Read the model definition and answer for the solid it produces. Units are mm, in the model's axes. A direction names the side the tool comes from. Coordinates: 2 decimals unless noted, no trailing zeros. Loops run counter-clockwise (first coordinate to the right, second up) from the corner with the lowest first, then second, coordinate; pieces in that order, holes last. Notation, with made-up numbers: M 40.5,18.5 L 79.5,18.5 A20 ccw 79.5,55.5 Z; hole C 0.25,15 d8. An arc over 180 degrees is marked long. One line per item, written item: value. Start each with the question number.
```python
from build123d import *

# Parameters (mm, degrees)
CROQUIS3_R            = 2.49
CORTAR_EXTRUIR1_DEPTH = 18
CROQUIS4_R            = 1.5
CORTAR_EXTRUIR2_DEPTH = 3


with BuildPart() as part:
    # Croquis2 → Revolución1 (revolve)
    with BuildSketch(Plane.XY, mode=Mode.PRIVATE) as revoluci_n1_sk:
        Polygon((0, 0), (-6, 0), (-6, 2), (-5, 2), (-5, 18), (-6, 18), (-6, 20), (0, 20), align=None)
    revolve(revoluci_n1_sk.sketch.rotate(Axis((0, 0, 0), (0, 1, 0)), 270), axis=Axis((0, 0, 0), (0, 1, 0)))

    # Croquis3 → Cortar-Extruir1 (cut)
    with BuildSketch(Plane.XZ):
        with Locations(Location((0, 0, 0), (0, 0, 270))):
            Circle(CROQUIS3_R)
    extrude(amount=-CORTAR_EXTRUIR1_DEPTH, mode=Mode.SUBTRACT)

    # Croquis4 → Cortar-Extruir2 (cut)
    with BuildSketch(Plane(origin=(5, 0, 0), x_dir=(0, 0, -1), z_dir=(1, 0, 0))):
        with Locations((0, 10)):
            Circle(CROQUIS4_R)
    extrude(amount=-CORTAR_EXTRUIR2_DEPTH, mode=Mode.SUBTRACT)


solid = part.part
```
1) Section B-B (z = 5.25) is taken. Determine the outline of the cut face in (x, y).
2) Flat-ended cylindrical pins translate along their axes: pin 1 (3 mm diameter, centred on y = 12.5, z = 3, fed in from -X); pin 2 (5 mm diameter, centred on y = 10.5, z = 2.5, fed in from +X); pin 3 (2.5 mm diameter, centred on y = 10, z = 0, fed in from +X). Find the tip coordinate at first contact, or state that the pin passes through.
3) A tool of negligible diameter and unlimited length cuts with its end or side. For faces 4 (the face through (0, 18, 0)), 5 (the face through (-1.802, 19.014, -5.723)), 6 (the face through (-4, 10, -3)), 7 (the face through (3.5, 9.1, 1.2)), from which of +Z, -Z, +X, -X, +Y, -Y can it reach the whole face along a straight path? Write none if from no direction.
4) Section D-D (z = 0) is taken. Determine the outline of the cut face in (x, y).
5) Consider line 1 along Y through (x, z) = (3.05, 0); line 2 along Y through (x, z) = (5, -1.5); line 3 along X through (y, z) = (6, 0). Determine where each line is inside the solid, lowest interval first.
6) Section A-A (x = 0) is taken. Determine the outline of the cut face in (y, z).
7) Section C-C (y = 5.25) is taken. Determine the outline of the cut face in (x, z).
8) For a pull along Z with two mould halves and no side action, classify faces 1 (the face through (-1.802, 1.014, -5.723)), 2 (the face through (-4, 18, -4)), 3 (the face through (-2.43, 8.87, 0.54)) as released by +Z, released by -Z, zero draft, split by the parting line, or undercut.
Results found:
1. outline: M -2.9,0 L 2.9,0 L 2.9,2 L -2.9,2 Z; M -2.9,18 L 2.9,18 L 2.9,20 L -2.9,20 Z
2. pin 1: stops at x = -4.77
2. pin 2: stops at x = 5
2. pin 3: stops at x = -2.15
3. face 4: -Y
3. face 5: +Y, -Y
3. face 6: none
3. face 7: +X
4. outline: M -6,0 L -2.49,0 L -2.49,18 L 2.49,18 L 2.49,11.5 L 5,11.5 L 5,18 L 6,18 L 6,20 L -6,20 L -6,18 L -5,18 L -5,2 L -6,2 Z; M 2.49,0 L 6,0 L 6,2 L 5,2 L 5,8.5 L 2.49,8.5 Z
5. line 1: y = 0 to 8.5, 11.5 to 20
5. line 2: y = 0 to 2, 18 to 20
5. line 3: x = -5 to -2.49, 2.49 to 5
6. outline: M 0,-6 L 2,-6 L 2,-5 L 18,-5 L 18,-6 L 20,-6 L 20,6 L 18,6 L 18,5 L 2,5 L 2,6 L 0,6 L 0,2.49 L 18,2.49 L 18,-2.49 L 0,-2.49 Z
7. outline: C 0,0 d10; hole C 0,0 d4.98
8. face 1: split by the parting line
8. face 2: zero draft
8. face 3: undercut
